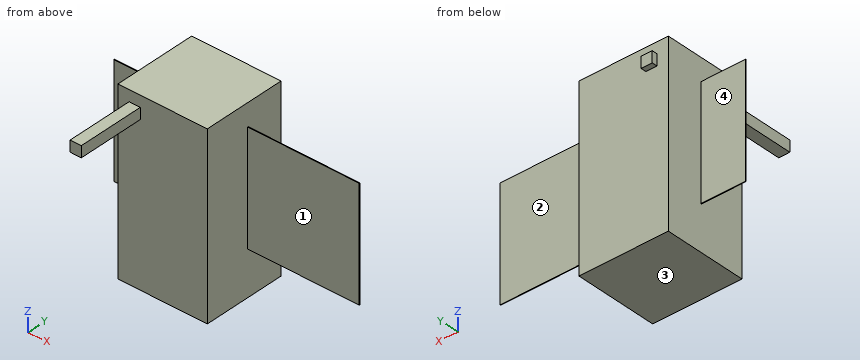
from build123d import *

# Parameters (mm, degrees)
F0_W          = 20.32
F0_H          = 40.64
F1_DEPTH      = 19.05
F2_W          = 0.1524
F2_H          = 25.4
F3_DEPTH      = 25.4
F3_DEPTH_BACK = 30.48
F4_W          = 2.54
F4_H          = 2.54
F5_DEPTH      = 15.24
F5_DEPTH_BACK = 20.32


with BuildPart() as f1:
    # F0 (on Front) → F1 (new body)
    with BuildSketch(Plane.XZ):
        with Locations((10.16, 20.32)):
            Rectangle(F0_W, F0_H)
    extrude(amount=F1_DEPTH)

    # F2 (on face) → F3 (join, two sides)
    with BuildSketch(Plane.YZ.offset(20.32)) as f3_sk:
        with Locations((-8.5344, 22.86)):
            Rectangle(F2_W, F2_H)
    extrude(amount=F3_DEPTH)
    extrude(f3_sk.sketch, amount=-F3_DEPTH_BACK)

    # F4 (on face) → F5 (join, two sides)
    with BuildSketch(Plane.XZ.offset(19.05)) as f5_sk:
        with Locations((3.81, 36.83)):
            Rectangle(F4_W, F4_H)
    extrude(amount=F5_DEPTH)
    extrude(f5_sk.sketch, amount=-F5_DEPTH_BACK)


solid = f1.part
Check sheet for the modelled part. Datum: model origin and axes. Units: mm. Face numbers are marked on the shaded views. A direction names the side the tool comes from. Round coordinates to 2 decimals unless told otherwise and drop trailing zeros. Loops run counter-clockwise (first coordinate to the right, second up) from the corner with the lowest first, then second, coordinate; pieces in that order, holes last. Notation, with made-up numbers: (60.5, 88.25) -> (78.5, 88.25) arc R27 ccw to (78.5, 109.25) -> close; hole circle Ø2 at (37, -14). An arc over 180 degrees is marked (long way). Put each result on its own line as item: value. Start each with the question number.
1. Section check A-A (z = 34). Enter the section's corners in (x, y), plus the area to 3 significant figures.
2. Section check B-B (x = 21.5). Enter the section's corners in (y, z), plus the area to 3 significant figures.
3. Gauge pin test, flat ends, axial feed: pin 1 (3 mm diameter, centred on x = 1, z = 22.5, fed in from +Y); pin 2 (0.8 mm diameter, centred on y = -25.5, z = 37, fed in from -X); pin 3 (0.6 mm diameter, centred on y = 0.5, z = 37, fed in from +X). Record the tip position at first contact, or that the pin passes through.
4. Access from +Z, -Z, +X, -X, +Y, -Y to the whole of each face (thin tool, end or side, straight path). Record for the marked faces 1, 2, 3 and 4.
5. Section check C-C (y = -10.5). Enter the section's corners in (x, z).
6. Scan lines: probe 1 along X at (y, z) = (-15, 7.5); probe 2 along Y at (x, z) = (5.5, 28); probe 3 along Y at (x, z) = (-7, 22). Record each from-to range of solid material in increasing order.
Findings:
1. outline: (-10.16, -8.61) -> (0, -8.61) -> (0, -19.05) -> (20.32, -19.05) -> (20.32, -8.61) -> (45.72, -8.61) -> (45.72, -8.46) -> (20.32, -8.46) -> (20.32, 0) -> (0, 0) -> (0, -8.46) -> (-10.16, -8.46) -> close
1. area: 393 mm^2
2. outline: (-8.61, 10.16) -> (-8.46, 10.16) -> (-8.46, 35.56) -> (-8.61, 35.56) -> close
2. area: 3.87 mm^2
3. pin 1: stops at y = 0
3. pin 2: stops at x = 2.54
3. pin 3: stops at x = 5.08
4. face 1: +Z, -Z, +X, -Y
4. face 2: +Z, -Z, +X, +Y
4. face 3: -Z, +X, -X, +Y, -Y
4. face 4: +Z, -Z, -X, +Y
5. outline: (0, 0) -> (20.32, 0) -> (20.32, 40.64) -> (0, 40.64) -> close
6. probe 1: x = 0 to 20.32
6. probe 2: y = -19.05 to 0
6. probe 3: y = -8.61 to -8.46
